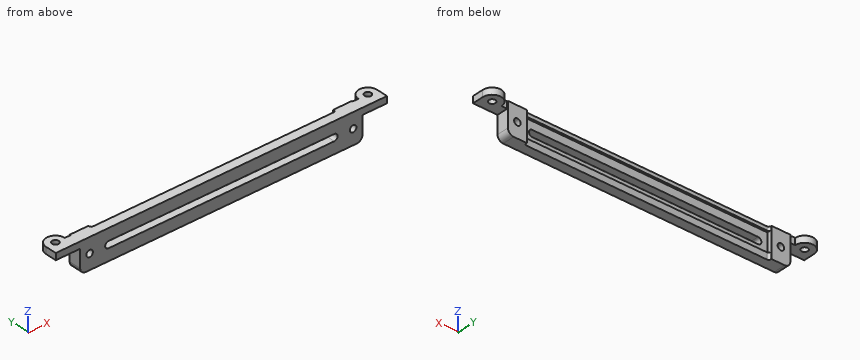
from build123d import *

# Parameters (mm, degrees)
SKETCH1_R           = 1.75
BOSS_EXTRUDE1_DEPTH = 4
SKETCH2_W           = 130
SKETCH2_H           = 10.5
SKETCH2_R           = 1.75
BOSS_EXTRUDE2_DEPTH = 1
SKETCH3_R           = 1.75
BOSS_EXTRUDE3_DEPTH = 1.5
FILLET1_R           = 1
SKETCH4_R           = 1.75
BOSS_EXTRUDE4_DEPTH = 3.5


with BuildPart() as part:
    # Sketch1 → Boss-Extrude1 (new body)
    with BuildSketch(Plane(origin=(0, 0, 0), x_dir=(1, 0, 0), z_dir=(0, 1, 0))):
        with BuildLine():
            Line((-75, -8), (75, -8))
            Line((75, -8), (75, 5))
            ThreePointArc((75, 5), (74.121320344, 7.121320344), (72, 8))
            Line((72, 8), (-72, 8))
            ThreePointArc((-72, 8), (-74.121320344, 7.121320344), (-75, 5))
            Line((-75, 5), (-75, -8))
        make_face()
        with Locations(Location((-70, 0, 0), (0, 0, 270))):
            Circle(SKETCH1_R, mode=Mode.SUBTRACT)
        with BuildLine():
            ThreePointArc((61.75, 0), (61.237436867, -1.237436867), (60, -1.75))
            Line((60, -1.75), (-60, -1.75))
            ThreePointArc((-60, -1.75), (-61.75, 0), (-60, 1.75))
            Line((-60, 1.75), (60, 1.75))
            ThreePointArc((60, 1.75), (61.237436867, 1.237436867), (61.75, 0))
        make_face(mode=Mode.SUBTRACT)
        with Locations(Location((70, 0, 0), (0, 0, 270))):
            Circle(SKETCH1_R, mode=Mode.SUBTRACT)
    extrude(amount=BOSS_EXTRUDE1_DEPTH)

    # Sketch2 → Boss-Extrude2 (add)
    with BuildSketch(Plane(origin=(0, 4, 0), x_dir=(1, 0, 0), z_dir=(0, 1, 0))):
        with BuildLine():
            Line((-75, -8), (75, -8))
            Line((75, -8), (75, 5))
            ThreePointArc((75, 5), (74.121320344, 7.121320344), (72, 8))
            Line((72, 8), (-72, 8))
            ThreePointArc((-72, 8), (-74.121320344, 7.121320344), (-75, 5))
            Line((-75, 5), (-75, -8))
        make_face()
        with Locations((0, -0.75)):
            Rectangle(SKETCH2_W, SKETCH2_H, mode=Mode.SUBTRACT)
        with Locations(Location((-70, 0, 0), (0, 0, 270))):
            Circle(SKETCH2_R, mode=Mode.SUBTRACT)
        with Locations(Location((70, 0, 0), (0, 0, 270))):
            Circle(SKETCH2_R, mode=Mode.SUBTRACT)
    extrude(amount=BOSS_EXTRUDE2_DEPTH)

    # Sketch3 → Boss-Extrude3 (add)
    # profile 1 of 2: a face of its own
    with BuildSketch(Plane(origin=(0, 5, 0), x_dir=(1, 0, 0), z_dir=(0, 1, 0))):
        with BuildLine():
            Line((65, 4.5), (65, 8))
            Line((65, 8), (72, 8))
            ThreePointArc((72, 8), (74.121320344, 7.121320344), (75, 5))
            Line((75, 5), (75, -8))
            Line((75, -8), (65, -8))
            Line((65, -8), (65, -6))
            Line((65, -6), (65, 4.5))
        make_face()
        with Locations(Location((70, 0, 0), (0, 0, 270))):
            Circle(SKETCH3_R, mode=Mode.SUBTRACT)
    # profile 2 of 2: a face of its own
    with BuildSketch(Plane(origin=(0, 5, 0), x_dir=(1, 0, 0), z_dir=(0, 1, 0))):
        with BuildLine():
            Line((-65, 4.5), (-65, 8))
            Line((-65, 8), (-72, 8))
            ThreePointArc((-72, 8), (-74.121320344, 7.121320344), (-75, 5))
            Line((-75, 5), (-75, -8))
            Line((-75, -8), (-65, -8))
            Line((-65, -8), (-65, -6))
            Line((-65, -6), (-65, 4.5))
        make_face()
        with Locations(Location((-70, 0, 0), (0, 0, 270))):
            Circle(SKETCH3_R, mode=Mode.SUBTRACT)
    extrude(amount=BOSS_EXTRUDE3_DEPTH)

    # Fillet1
    fillet1_edges = [part.edges().sort_by_distance(p)[0] for p in [
        (-65, 5, 7),
        (65, 5, 7),
        (65, 5, -6.25),
        (-65, 5, -6.25),
    ]]
    fillet(fillet1_edges, radius=FILLET1_R)

    # Sketch4 → Boss-Extrude4 (add)
    # profile 1 of 2: a face of its own
    with BuildSketch(Plane.XY.offset(8)):
        with BuildLine():
            Line((-88, 0), (-75, 0))
            Line((-75, 0), (-75, 6))
            Line((-75, 6), (-78, 6))
            ThreePointArc((-78, 6), (-83, 11), (-88, 6))
            Line((-88, 6), (-88, 0))
        make_face()
        with Locations((-83, 6)):
            Circle(SKETCH4_R, mode=Mode.SUBTRACT)
    # profile 2 of 2: a face of its own
    with BuildSketch(Plane.XY.offset(8)):
        with BuildLine():
            Line((78, 6), (75, 6))
            Line((75, 6), (75, 0))
            Line((75, 0), (88, 0))
            Line((88, 0), (88, 6))
            ThreePointArc((88, 6), (83, 11), (78, 6))
        make_face()
        with Locations((83, 6)):
            Circle(SKETCH4_R, mode=Mode.SUBTRACT)
    extrude(amount=-BOSS_EXTRUDE4_DEPTH)


solid = part.part
Verification items for the finished model (mm, model axes). Coordinates: 2 decimals unless noted, no trailing zeros. Loops run counter-clockwise (first coordinate to the right, second up) from the corner with the lowest first, then second, coordinate; pieces in that order, holes last. Notation, with made-up numbers: (-5.5, 51.25) -> (4.5, 51.25) arc R26 ccw to (4.5, 69.25) -> close; hole circle Ø6 at (57, 54). An arc over 180 degrees is marked (long way). Answer as a JSON object with one key per item and string values. Group by question number.
Item 1: Sectioned sample at A-A on x = -83. Record the boundary of the cut face in (y, z).
Item 2: Sectioned sample at B-B on y = 1.5. Record the boundary of the cut face in (x, z).
Item 3: Depth check by flat-ended pin: pin 1 (2 mm diameter, centred on x = 83, y = 6, fed in from -Z); pin 2 (5.5 mm diameter, centred on x = -70, z = 0, fed in from +Y); pin 3 (1.8 mm diameter, centred on x = 19.5, z = -6.5, fed in from +Y); pin 4 (1 mm diameter, centred on y = 4, z = -3, fed in from -X). Enter the tip coordinate at first touch or a pass-through.
Item 4: Sectioned sample at C-C on x = 17.5. Record the boundary of the cut face in (y, z).
Item 5: Scan lines: probe 1 along X at (y, z) = (4.5, 0); probe 2 along X at (y, z) = (3.25, 0); probe 3 along Z at (x, y) = (-32.5, 0.5). Record each from-to range of solid material in increasing order.
Evaluation:
{
 "1": {"outline": "(0, 4.5) -> (4.25, 4.5) -> (4.25, 8) -> (0, 8) -> close; (7.75, 4.5) -> (11, 4.5) -> (11, 8) -> (7.75, 8) -> close"},
 "2": {"outline": "(-88, 4.5) -> (-75, 4.5) -> (-75, -5) arc R3 ccw to (-72, -8) -> (72, -8) arc R3 ccw to (75, -5) -> (75, 4.5) -> (88, 4.5) -> (88, 8) -> (-88, 8) -> close; hole circle Ø3.5 at (-70, 0); hole (-60, -1.75) -> (60, -1.75) arc R1.75 ccw to (60, 1.75) -> (-60, 1.75) arc R1.75 ccw to start; hole circle Ø3.5 at (70, 0)"},
 "3": {"pin 1": "passes through", "pin 2": "stops at y = 6.5", "pin 3": "stops at y = 5", "pin 4": "stops at x = -75"},
 "4": {"outline": "(0, -8) -> (5, -8) -> (5, -4.5) -> (4, -4.5) -> (4, -1.75) -> (0, -1.75) -> close; (0, 1.75) -> (4, 1.75) -> (4, 6) -> (5, 6) -> (5, 8) -> (0, 8) -> close"},
 "5": {"probe 1": "x = -75 to -71.75, -68.25 to -65, 65 to 68.25, 71.75 to 75", "probe 2": "x = -75 to -71.75, -68.25 to -61.75, 61.75 to 68.25, 71.75 to 75", "probe 3": "z = -8 to -1.75, 1.75 to 8"}
}
